Can you work these out from the model? Positions are in its coordinate system, mm. Face numbers are marked on the shaded views. A direction names the side the tool comes from. Coordinates: 2 decimals unless noted, no trailing zeros. Loops run counter-clockwise (first coordinate to the right, second up) from the corner with the lowest first, then second, coordinate; pieces in that order, holes last. Notation, with made-up numbers: (46, -30.5) -> (72, -30.5) arc R20 cw to (72, -5.5) -> close; hole circle Ø9 at (-27, 16). An arc over 180 degrees is marked (long way). Use one line per item in the form item = value. Start each with the question number.
(1) Imagine slicing it at B-B (y = 2). List the corners of the cut face in (x, z) for me.
(2) On a 3-axis mill with a long thin cutter (end or side, diameter ignored), from which of +Z, -Z, +X, -X, +Y, -Y can I reach the whole of each face in a straight line? I mean the marked faces 1 and 2. Say none if no direction works.
(3) Imagine slicing it at C-C (z = 2.5). List the corners of the cut face in (x, y) for me, plus the area to 3 significant figures.
(4) I'm going to push flat-ended pins straight in: pin 1 (5 mm diameter, centred on x = 1, y = 6.5, fed in from -Z); pin 2 (2 mm diameter, centred on x = 5.5, z = 5.5, fed in from -Y); pin 3 (4 mm diameter, centred on y = 2, z = 7, fed in from +X). Where does each tip first touch, or does it pass through?
(5) I need wall thicknesses on line 1 (X direction, y = 2.75, z = 4.5); line 2 (X direction, y = 6, z = 5.75). Which ranges of each line are inside material? Lowest first, please. Write a range as [from, to].
(6) Imagine slicing it at D-D (x = 4.5). List the corners of the cut face in (y, z) for me, plus the area to 3 significant figures.
(7) Imagine slicing it at A-A (x = 6.5). List the corners of the cut face in (y, z) for me.
```python
from build123d import *

# Parameters (mm, degrees)
F1_DEPTH = 3
F2_DEPTH = 9
F7_DEPTH = 5.1971524227


with BuildPart() as f1:
    # F0 (on Top) → F1 (new body)
    with BuildSketch(Plane.XY):
        Polygon((0, 10), (0, 0), (3, 0), (3, 5), (9, 8), (9, 10), align=None)
        Polygon((3, 5), (3, 0), (9, 0), (9, 8), align=None)
    extrude(amount=F1_DEPTH)

    # F0 (on Top) → F2 (join)
    with BuildSketch(Plane.XY):
        Polygon((0, 10), (0, 0), (3, 0), (3, 5), (9, 8), (9, 10), align=None)
    extrude(amount=F2_DEPTH)

    # F6 (on 3pt) → F7 (cut, through all)
    with BuildSketch(Plane(origin=(3, -3, 3), x_dir=(0.4082482905, 0.8164965809, 0.4082482905), z_dir=(0.5773502692, -0.5773502692, 0.5773502692))):
        Polygon((7.3484692283, -4.2426406871), (3.6742346142, -2.1213203436), (3.6742346142, -6.3639610307), align=None)
    extrude(amount=F7_DEPTH, mode=Mode.SUBTRACT)


solid = f1.part
```
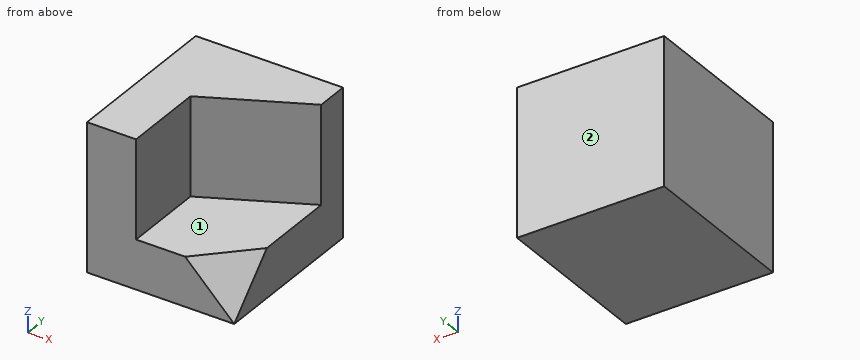
Worked out:
q1.outline = (0, 0) -> (9, 0) -> (9, 2) -> (8, 3) -> (3, 3) -> (3, 9) -> (0, 9) -> close
q2.face_1 = +Z, +X, -Y
q2.face_2 = +Z, -Z, +X, -X, +Y
q3.outline = (0, 0) -> (6.5, 0) -> (9, 2.5) -> (9, 10) -> (0, 10) -> close
q3.area = 86.9 mm2
q4.pin_1 = 0
q4.pin_2 = 5.75
q4.pin_3 = 3
q5.line_1 = [0, 3]
q5.line_2 = [0, 5]
q6.outline = (0, 0) -> (10, 0) -> (10, 9) -> (5.75, 9) -> (5.75, 3) -> (0, 3) -> close
q6.area = 55.5 mm2
q7.outline = (0, 0) -> (10, 0) -> (10, 9) -> (6.75, 9) -> (6.75, 3) -> (0.5, 3) -> (0, 2.5) -> close
